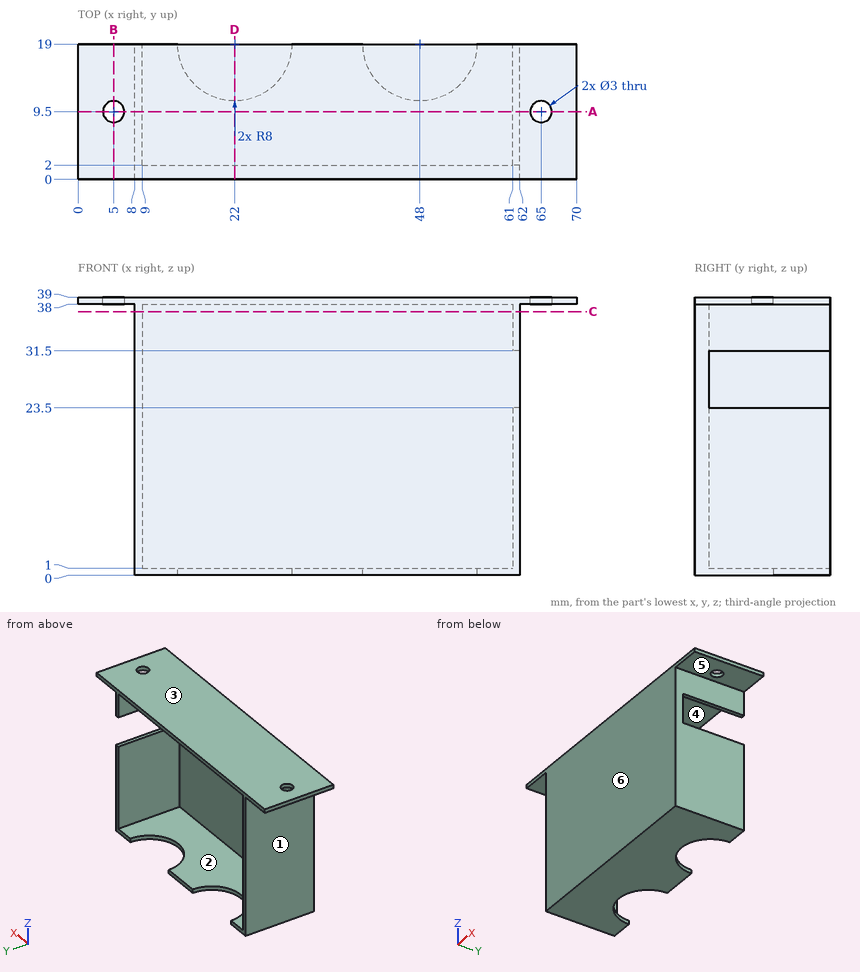
Geometry check sheet. Reference: drawing and pictorial views, mm from the part's lowest x, y, z. A direction names the side the tool comes from. Round coordinates to 2 decimals unless told otherwise and drop trailing zeros. Write each loop counter-clockwise with the first axis right and the second up, starting at its lowest first coordinate (ties: lowest second). Pieces come first, ordered by that corner, then holes.
1. Section check C-C on z = 37. Enter the section's corners in (x, y), plus the area to 3 significant figures.
2. Section check A-A on y = 9.5. Enter the section's corners in (x, z).
3. Scan lines: L1, parallel to X at y = 2.75, z = 19; L2, parallel to Z at x = 51.5, y = 9.5; L3, parallel to Y at x = 5, z = 38.3. Record each from-to range of solid material in increasing order.
4. Section check B-B on x = 5. Enter the section's corners in (y, z).
5. Draft check along X on the marked faces 1, 2 and 3. Enter one of: +X half, -X half, draft (parallel to the pull), parting line (faces both ways), or undercut.
6. Section check D-D on x = 22. Enter the section's corners in (y, z), plus the area to 3 significant figures.
7. Gauge pin test, flat ends, axial feed: P1, Ø1.5, axis at y = 2.5, z = 31.5, coming from the +X side; P2, Ø1.5, axis at x = 43, z = 12.5, coming from the +Y side; P3, Ø5, axis at y = 12, z = 26.5, coming from the +X side. Record the tip position at first contact, or that the pin passes through.
8. Access from +Z, -Z, +X, -X, +Y, -Y to the whole of each face (thin tool, end or side, straight path). Record for the marked faces 4, 5 and 6.
Answer:
1. outline: (8, 0) - (62, 0) - (62, 19) - (61, 19) - (61, 2) - (9, 2) - (9, 19) - (8, 19) - close
1. area: 142 mm2
2. outline: (0, 38) - (3.5, 38) - (3.5, 39) - (0, 39) - close; (6.5, 38) - (8, 38) - (8, 0) - (62, 0) - (62, 23.5) - (61, 23.5) - (61, 1) - (9, 1) - (9, 38) - (61, 38) - (61, 31.5) - (62, 31.5) - (62, 38) - (63.5, 38) - (63.5, 39) - (6.5, 39) - close; (66.5, 38) - (70, 38) - (70, 39) - (66.5, 39) - close
3. L1: x = 8 to 9, 61 to 62
3. L2: z = 0 to 1, 38 to 39
3. L3: y = 0 to 8, 11 to 19
4. outline: (0, 38) - (8, 38) - (8, 39) - (0, 39) - close; (11, 38) - (19, 38) - (19, 39) - (11, 39) - close
5. face 1: -X half
5. face 2: undercut
5. face 3: draft
6. outline: (0, 0) - (11, 0) - (11, 1) - (2, 1) - (2, 38) - (19, 38) - (19, 39) - (0, 39) - close
6. area: 104 mm2
7. P1: stops at x = 62
7. P2: stops at y = 2
7. P3: stops at x = 9
8. face 4: +Y
8. face 5: -Z, +X, +Y, -Y
8. face 6: +Z, -Z, +X, -X, -Y
